Work out the finished part from the listing and answer in its coordinate system (mm). Face numbers are marked on the shaded views. A direction names the side the tool comes from. Coordinates: 2 decimals unless noted, no trailing zeros. Order: outer loops, then holes, each group sorted by start corner. A loop starts at its lowest first (then second) coordinate and runs counter-clockwise, first axis right, second up. Notation, with made-up numbers: M 39,-6.5 L 58,-6.5 A32 ccw 58,23.5 Z; hole C -28.5,-10.75 d2. An arc over 180 degrees is marked long. Use a Markdown table: item, result.
from build123d import *

# Parameters (mm, degrees)
SKETCH1_R           = 71.4375
BOSS_EXTRUDE1_DEPTH = 188.4934
SKETCH2_R           = 2.308225
BOSS_EXTRUDE2_DEPTH = 25.4
BOSS_EXTRUDE3_DEPTH = 57.15
SKETCH4_W           = 130.175
SKETCH4_H           = 101.6
SKETCH4_R           = 4.3688
BOSS_EXTRUDE4_DEPTH = 76.2


with BuildPart() as part:
    # Sketch1 → Boss-Extrude1 (new body)
    with BuildSketch(Plane.XY):
        Circle(SKETCH1_R)
    extrude(amount=BOSS_EXTRUDE1_DEPTH)

    # Sketch2 → Boss-Extrude2 (add)
    with BuildSketch(Plane.XY.offset(188.4934)):
        with Locations((-46.0375, 46.0375)):
            Circle(SKETCH2_R)
        with Locations((-46.0375, -46.0375)):
            Circle(SKETCH2_R)
        with Locations((46.0375, -46.0375)):
            Circle(SKETCH2_R)
        with Locations((46.0375, 46.0375)):
            Circle(SKETCH2_R)
    extrude(amount=BOSS_EXTRUDE2_DEPTH)

    # Sketch3 → Boss-Extrude3 (add)
    with BuildSketch(Plane.XY.offset(188.4934)):
        with BuildLine():
            Line((-3.062675504, 5.5626), (3.062675504, 5.5626))
            ThreePointArc((3.062675504, 5.5626), (0, -6.35), (-3.062675504, 5.5626))
        make_face()
    extrude(amount=BOSS_EXTRUDE3_DEPTH)

    # Sketch4 → Boss-Extrude4 (add)
    with BuildSketch(Plane(origin=(0, 0, 0), x_dir=(1, 0, 0), z_dir=(0, 1, 0))):
        with Locations((0, -86.8934)):
            Rectangle(SKETCH4_W, SKETCH4_H)
        with Locations((-53.975, -121.8184)):
            Circle(SKETCH4_R, mode=Mode.SUBTRACT)
        with Locations((53.975, -121.8184)):
            Circle(SKETCH4_R, mode=Mode.SUBTRACT)
        with Locations((-53.975, -51.9684)):
            Circle(SKETCH4_R, mode=Mode.SUBTRACT)
        with Locations((53.975, -51.9684)):
            Circle(SKETCH4_R, mode=Mode.SUBTRACT)
    extrude(amount=-BOSS_EXTRUDE4_DEPTH)


solid = part.part
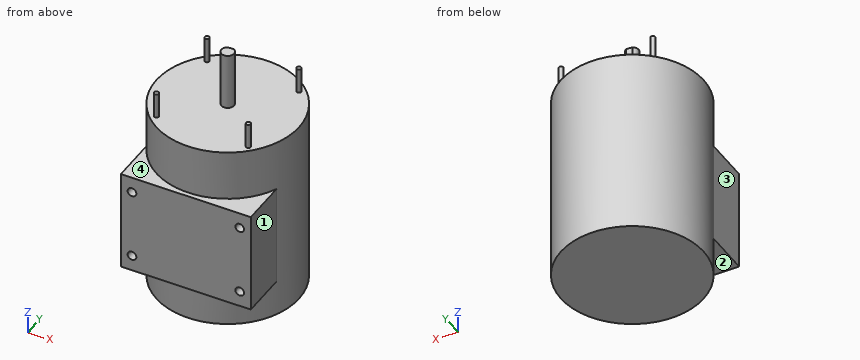
1. Section A-A on y = 0 is taken. Determine the outline of the cut face in (x, z).
Answers below:
| item | result |
|---|---|
| outline | M -71.44,0 L 71.44,0 L 71.44,188.49 L 6.35,188.49 L 6.35,245.64 L -6.35,245.64 L -6.35,188.49 L -71.44,188.49 Z |
2. For the marked faces 1, 2, 3 and 4, determine the directions among +Z, -Z, +X, -X, +Y, -Y from which every point of the face is accessible in a straight line to the end or side of a thin tool.
Answers below:
| item | result |
|---|---|
| face 1 | +Z, -Z, +X, -Y |
| face 2 | -Z, -Y |
| face 3 | +Z, -Z, -X, -Y |
| face 4 | +Z, -Y |
3. Flat-ended cylindrical pins translate along their axes: P1, Ø2.5, axis at x = -47, y = 46.5, coming from the +Z side; P2, Ø12, axis at x = -30.5, y = -2, coming from the +Z side; P3, Ø1.8, axis at x = -0.5, z = 230, coming from the +Y side. Find the tip coordinate at first contact, or state that the pin passes through.
Answers below:
| item | result |
|---|---|
| P1 | z = 213.89 |
| P2 | z = 188.49 |
| P3 | y = 5.56 |
4. Section D-D on z = 150.5 is taken. Determine the outline of the cut face in (x, y) (1 decimal).
Answers below:
| item | result |
|---|---|
| outline | C 0,0 d142.9 |
5. Find the intervals of material crossed by probe 1 along Z at (x, y) = (40, -18); probe 2 along Y at (x, z) = (-56.5, 153.5); probe 3 along X at (y, z) = (-65, 135.5), in increasing order.
Answers below:
| item | result |
|---|---|
| probe 1 | 0 to 188.49 |
| probe 2 | -43.72 to 43.72 |
| probe 3 | -65.09 to 65.09 |
6. Section B-B on z = 200 is taken. Determine the outline of the cut face in (x, y).
Answers below:
| item | result |
|---|---|
| outline | C -46.04,-46.04 d4.62; C -46.04,46.04 d4.62; M -3.06,5.56 A6.35 ccw long 3.06,5.56 Z; C 46.04,-46.04 d4.62; C 46.04,46.04 d4.62 |
7. Section C-C on x = 0 is taken. Determine the outline of the cut face in (y, z), then the cut area to 3 significant figures.
Answers below:
| item | result |
|---|---|
| outline | M -76.2,36.09 L -71.44,36.09 L -71.44,0 L 71.44,0 L 71.44,188.49 L 5.56,188.49 L 5.56,245.64 L -6.35,245.64 L -6.35,188.49 L -71.44,188.49 L -71.44,137.69 L -76.2,137.69 Z |
| area | 28,100 mm² |
